Check sheet for the modelled part. Datum: model origin and axes. Units: mm. A direction names the side the tool comes from. Give positions to 0.01 mm unless a question says otherwise; leave off trailing zeros. Write each loop counter-clockwise with the first axis right and the second up, starting at its lowest first coordinate (ties: lowest second). Pieces come first, ordered by that corner, then holes.
from build123d import *

# Parameters (mm, degrees)
SKETCH_1_W          = 250
SKETCH_1_H          = 156
SKETCH_1_W_2        = 226
SKETCH_1_H_2        = 128
EXTRUDE_1_DEPTH     = 8
SKETCH_2_W          = 235.5
SKETCH_2_H          = 139.5
CUT_EXTRUDE_3_DEPTH = 6
SKETCH_11_W         = 250
SKETCH_11_H         = 8
EXTRUDE_3_DEPTH     = 3.75
CUT_EXTRUDE_4_DEPTH = 10
SKETCH_13_R         = 2
CUT_EXTRUDE_5_DEPTH = 6
SKETCH_14_W         = 6.25
SKETCH_14_H         = 17.2
CUT_EXTRUDE_6_DEPTH = 1.5
SKETCH_16_W         = 3.85
SKETCH_16_H         = 17.2
CUT_EXTRUDE_8_DEPTH = 1.5


with BuildPart() as part:
    # 草图1 → 凸台-拉伸1 (new body)
    with BuildSketch(Plane(origin=(0, 0, 0), x_dir=(1, 0, 0), z_dir=(0, 1, 0))):
        with Locations((25.659327926, -14.898030127)):
            Rectangle(SKETCH_1_W, SKETCH_1_H)
        with Locations((25.659327926, -14.898030127)):
            Rectangle(SKETCH_1_W_2, SKETCH_1_H_2, mode=Mode.SUBTRACT)
    extrude(amount=EXTRUDE_1_DEPTH)

    # 草图2 → 切除-拉伸3 (cut)
    with BuildSketch(Plane.XZ):
        with Locations((24.659327926, 12.898030127)):
            Rectangle(SKETCH_2_W, SKETCH_2_H)
    extrude(amount=-CUT_EXTRUDE_3_DEPTH, mode=Mode.SUBTRACT)

    # 草图11 → 凸台-拉伸3 (add)
    with BuildSketch(Plane(origin=(0, 0, -63.101969873), x_dir=(-1, 0, 0), z_dir=(0, 0, -1))):
        with Locations((-25.659327926, 4)):
            Rectangle(SKETCH_11_W, SKETCH_11_H)
    extrude(amount=EXTRUDE_3_DEPTH)

    # 草图12 → 切除-拉伸4 (cut)
    with BuildSketch(Plane.XZ):
        with BuildLine():
            Line((-89.340672074, 92.898030127), (-99.340672074, 92.898030127))
            Line((-99.340672074, 92.898030127), (-99.340672074, 82.898030127))
            ThreePointArc((-99.340672074, 82.898030127), (-96.411739886, 89.969097939), (-89.340672074, 92.898030127))
        make_face()
        with BuildLine():
            Line((-99.340672074, -56.851969873), (-99.340672074, -66.851969873))
            Line((-99.340672074, -66.851969873), (-89.340672074, -66.851969873))
            ThreePointArc((-89.340672074, -66.851969873), (-96.411739886, -63.923037684), (-99.340672074, -56.851969873))
        make_face()
        with BuildLine():
            Line((140.659327926, -66.851969873), (150.659327926, -66.851969873))
            Line((150.659327926, -66.851969873), (150.659327926, -56.851969873))
            ThreePointArc((150.659327926, -56.851969873), (147.730395738, -63.923037684), (140.659327926, -66.851969873))
        make_face()
        with BuildLine():
            Line((150.659327926, 82.898030127), (150.659327926, 92.898030127))
            Line((150.659327926, 92.898030127), (140.659327926, 92.898030127))
            ThreePointArc((140.659327926, 92.898030127), (147.730395738, 89.969097939), (150.659327926, 82.898030127))
        make_face()
    extrude(amount=-CUT_EXTRUDE_4_DEPTH, mode=Mode.SUBTRACT)

    # 草图13 → 切除-拉伸5 (cut)
    with BuildSketch(Plane.XZ):
        with Locations(Location((-86.340672074, 87.898030127, 0), (0, 0, 270))):
            Circle(SKETCH_13_R)
        with Locations(Location((137.659327926, 87.898030127, 0), (0, 0, 270))):
            Circle(SKETCH_13_R)
        with Locations(Location((137.659327926, -61.851969873, 0), (0, 0, 270))):
            Circle(SKETCH_13_R)
        with Locations(Location((-86.340672074, -61.851969873, 0), (0, 0, 270))):
            Circle(SKETCH_13_R)
    extrude(amount=-CUT_EXTRUDE_5_DEPTH, mode=Mode.SUBTRACT)

    # 草图14 → 切除-拉伸6 (cut)
    with BuildSketch(Plane.XZ):
        with Locations((-96.215672074, -19.101969873)):
            Rectangle(SKETCH_14_W, SKETCH_14_H)
    extrude(amount=-CUT_EXTRUDE_6_DEPTH, mode=Mode.SUBTRACT)

    # 草图16 → 切除-拉伸8 (cut)
    with BuildSketch(Plane.XZ.offset(-1.5)):
        with Locations((-95.015672074, -19.101969873)):
            Rectangle(SKETCH_16_W, SKETCH_16_H)
    extrude(amount=-CUT_EXTRUDE_8_DEPTH, mode=Mode.SUBTRACT)


solid = part.part
1) Access from +Z, -Z, +X, -X, +Y, -Y to the whole of each face (thin tool, end or side, straight path). Record for faces 4 (the flat face through (142.409, 3, 12)), 5 (the cylindrical face through (147.81, 3.94, -63.84)).
2) Sectioned sample at A-A on x = 20.5. Record the boundary of the cut face in (y, z), then the cut area to 3 significant figures.
3) Gauge pin test, flat ends, axial feed: pin 1 (5 mm diameter, centred on x = -86.34, z = -61.85, fed in from -Y); pin 2 (3.5 mm diameter, centred on x = -95.5, y = 1, fed in from +Z); pin 3 (1.2 mm diameter, centred on x = -98, z = -23.5, fed in from -Y); pin 4 (2 mm diameter, centred on x = 137, z = 88.5, fed in from -Y). Record the tip position at first contact, or that the pin passes through.
4) Draft check along Z on faces 1 (the cylindrical face through (147.7, 3.9, 90)), 2 (the flat face through (36, 0, 84)), 3 (the flat face through (23, 3, 82.648)). Enter one of: +Z half, -Z half, draft (parallel to the pull), parting line (faces both ways), or undercut.
5) Scan lines: L1, parallel to X at y = 3.25, z = -9; L2, parallel to X at y = 7.25, z = 73; L3, parallel to Z at x = 17, y = 4. Record each from-to range of solid material in increasing order.
6) Sectioned sample at C-C on y = 4.5. Record the boundary of the cut face in (x, z).
7) Sectioned sample at B-B on z = 70. Record the boundary of the cut face in (x, y).
Answers below:
1. face 4: -Y
1. face 5: -Z, +X, +Y, -Y
2. outline: (0, -66.85) - (8, -66.85) - (8, -49.1) - (6, -49.1) - (6, -56.85) - (0, -56.85) - close; (0, 82.65) - (6, 82.65) - (6, 78.9) - (8, 78.9) - (8, 92.9) - (0, 92.9) - close
2. area: 185 mm2
3. pin 1: stops at y = 0
3. pin 2: stops at z = 91.87
3. pin 3: stops at y = 1.5
3. pin 4: stops at y = 6
4. face 1: +Z half
4. face 2: draft
4. face 3: undercut
5. L1: x = -99.34 to -93.09, 142.41 to 150.66
5. L2: x = -99.34 to -87.34, 138.66 to 150.66
5. L3: z = -66.85 to -56.85, 82.65 to 92.9
6. outline: (-99.34, -56.85) arc R10 ccw to (-89.34, -66.85) - (140.66, -66.85) arc R10 ccw to (150.66, -56.85) - (150.66, 82.9) arc R10 ccw to (140.66, 92.9) - (-89.34, 92.9) arc R10 ccw to (-99.34, 82.9) - close; hole (-93.09, -56.85) - (142.41, -56.85) - (142.41, 82.65) - (-93.09, 82.65) - close; hole circle Ø4 at (-86.34, -61.85); hole circle Ø4 at (-86.34, 87.9); hole circle Ø4 at (137.66, -61.85); hole circle Ø4 at (137.66, 87.9)
7. outline: (-99.34, 0) - (-93.09, 0) - (-93.09, 6) - (-87.34, 6) - (-87.34, 8) - (-99.34, 8) - close; (138.66, 6) - (142.41, 6) - (142.41, 0) - (150.66, 0) - (150.66, 8) - (138.66, 8) - close
